Autodesk Fusion 360 part; units mm, degrees
sketch "Sketch1" plane through (0, 0, 0) normal (0, 0, 1) x (1, 0, 0)
  line L0 (89, 32) -> (-89, 32)
  line L1 (-89, 32) -> (-89, -32)
  line L2 (-89, -32) -> (89, -32)
  line L3 (89, -32) -> (89, 32)
  line L4 (89, 32) -> (-89, -32) construction
  line L5 (-89, 32) -> (89, -32) construction
  circle A0 centre (-57, 0) radius 11
  circle A1 centre (57, 0) radius 11
  dimension "d1" = 178
  dimension "d2" = 64
  dimension "d13" = 22
  dimension "d14" = 22
  dimension "d21" = 114
extrude "Extrude2" add sketch "Sketch1" along normal blind 19
fillet "Fillet3" radius 32 2 edges at (-89, -32, 9.5) (-89, 32, 9.5)
fillet "Fillet4" radius 32 2 edges at (89, -32, 9.5) (89, 32, 9.5)
sketch "Sketch2" plane through (0, 0, 19) normal (0, 0, 1) x (-1, 0, 0)
  arc A0 (-57, 32) -> (-57, -32) centre (-57, 0) ccw
  line L0 (-57, -32) -> (57, -32)
  arc A1 (57, -32) -> (57, 32) centre (57, 0) ccw
  line L1 (57, 32) -> (-57, 32)
  circle A2 centre (-57, 0) radius 11
  circle A3 centre (57, 0) radius 11
  line L2 (0, -32) -> (32, -32)
  line L3 (0, -32) -> (-32, -32)
  line L4 (32, -32) -> (32, 32)
  line L5 (-32, -32) -> (-32, 32)
  line L6 (32, 32) -> (19, 32)
  line L7 (-32, 32) -> (-19, 32)
  line L8 (19, 32) -> (19, -19)
  line L9 (-19, 32) -> (-19, -19)
  line L10 (19, -19) -> (-19, -19)
  dimension "d22" = 32
  dimension "d23" = 32
  dimension "d28" = 13
  dimension "d29" = 13
  dimension "d30" = 51
  dimension "d31" = 51
extrude "Extrude3" add sketch "Sketch2" along normal blind 45 contours L0 L1 L2 L3 L4 L5 L6 L7 L8 L9 L10
sketch "Sketch3" plane through (19, 0, 0) normal (-1, 0, 0) x (0, -1, 0)
  line L0 (-19, 19) -> (32, 19)
  line L1 (32, 19) -> (32, 64)
  line L2 (32, 64) -> (-19, 64)
  line L3 (-19, 64) -> (-19, 19)
sketch "Sketch4" plane through (0, 0, 0) normal (1, 0, 0) x (0, 1, 0)
  line L0 (19, 19) -> (-32, 19)
  line L1 (19, 19) -> (19, 64)
  line L2 (19, 64) -> (-32, 19)
  dimension "d34" = 51
  dimension "d35" = 45
extrude "Extrude4" add sketch "Sketch4" along normal mid plane 38
equation "d32 = 64 mm - 19 mm"
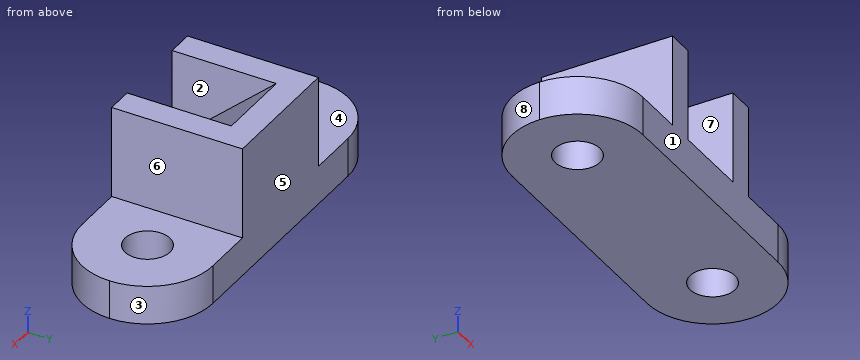
Source: CAD feature listing. Evaluate the final solid. Frame: model axes, mm. Face numbers are marked on the shaded views. A direction names the side the tool comes from. Coordinates: 2 decimals unless noted, no trailing zeros. Loops run counter-clockwise (first coordinate to the right, second up) from the corner with the lowest first, then second, coordinate; pieces in that order, holes last. Notation, with made-up numbers: (-25, 54) - (22, 54) arc R27 ccw to (22, 74) - close; hole circle Ø3 at (-15.75, 48.25). An arc over 180 degrees is marked (long way). One line per item, written item: value. Start each with the question number.
1. Section D-D (z = 56.5). Return the cut outline in (x, y), and give its area (3 significant figures).
2. Ray query, L1, parallel to Y at x = -57, z = 7; L2, parallel to X at y = 2, z = 8; L3, parallel to X at y = -18, z = 35.5. Return the intervals inside material, ascending.
3. Section B-B (z = 22). Return the cut outline in (x, y).
4. Set-up query: the marked faces 4, 5, 6, 7 and 8. Return all of +Z, -Z, +X, -X, +Y, -Y with unobstructed straight access to the full face (end or side cutting, diameter ignored); none if empty.
5. Section A-A (z = 8). State how many separate pieces and enclosed holes the cut face has, and give its area (3 significant figures).
6. Contact query for flat-ended pins moving along their axis: P1, Ø3, axis at x = 69, y = -16.5, coming from the -Z side; P2, Ø13.5, axis at y = -5.5, z = 52.5, coming from the +X side; P3, Ø5, axis at x = -2, y = -21.5, coming from the +Z side; P4, Ø2, axis at y = -9.5, z = 13, coming from the +X side. Output: stop coordinate, or through.
7. Mould query, pull axis X, two halves, no side actions, for the marked faces 1, 2 and 3. Classes: pulls with the +X half, pulls with the -X half, needs draft (parallel to the pull), parting line crosses it, or undercut.
8. Section C-C (y = -8.5). Return the cut outline in (x, z), and give its area (3 significant figures).
Verdict:
1. outline: (-32, -32) - (-19, -32) - (-19, 10.5) - (19, 10.5) - (19, -32) - (32, -32) - (32, 32) - (-32, 32) - close
1. area: 2,480 mm2
2. L1: y = -32 to -11, 11 to 32
2. L2: x = -88.94 to -67.82, -46.18 to 46.18, 67.82 to 88.94
2. L3: x = -32 to -19, 19 to 32
3. outline: (-32, -32) - (-19, -32) - (-19, -28.6) - (19, -28.6) - (19, -32) - (32, -32) - (32, 32) - (-32, 32) - close
4. face 4: +Z, -X, +Y, -Y
4. face 5: +Z, -Z, +X, -X, +Y
4. face 6: +Z, +X, +Y, -Y
4. face 7: +Z, -Y
4. face 8: +Z, -Z, -X, +Y
5. separate pieces: 1
5. enclosed holes: 2
5. area: 9,750 mm2
6. P1: stops at z = 0
6. P2: stops at x = 32
6. P3: stops at z = 30.47
6. P4: stops at x = 87.85
7. face 1: needs draft
7. face 2: undercut
7. face 3: pulls with the +X half
8. outline: (-87.85, 0) - (-63.98, 0) - (-63.98, 19) - (-87.85, 19) - close; (-50.02, 0) - (50.02, 0) - (50.02, 19) - (32, 19) - (32, 64) - (19, 64) - (19, 39.74) - (-19, 39.74) - (-19, 64) - (-32, 64) - (-32, 19) - (-50.02, 19) - close; (63.98, 0) - (87.85, 0) - (87.85, 19) - (63.98, 19) - close
8. area: 4,770 mm2
